Part model, mm, in its own coordinate system. Give positions to 0.01 mm unless a question says otherwise; leave off trailing zeros. Order: outer loops, then holes, each group sorted by start corner. A loop starts at its lowest first (then second) coordinate and runs counter-clockwise, first axis right, second up. Notation, with made-up numbers: (-18, -7.75) - (-10, -7.75) arc R15 cw to (-10, 18.25) - close; hole circle Ø6 at (66, 86). An arc over 180 degrees is marked (long way). One line per item, written item: value.
```python
from build123d import *
from OCP.BRepFilletAPI import BRepFilletAPI_MakeChamfer

# Parameters (mm, degrees)
BOSS_EXTRUDE1_DEPTH = 58.42
CHAMFER1_SIZE       = 6.35
CHAMFER1_SIZE2      = 6.020287439
CHAMFER1_SIZE2_2    = 11.16699707
CHAMFER2_SIZE       = 6.35
CHAMFER2_SIZE2      = 2.311210988
CHAMFER3_SIZE       = 6.35
CHAMFER3_SIZE_2     = 5.138982639
CHAMFER3_SIZE_3     = 2.835119985
CHAMFER3_SIZE_4     = 2.311210988


with BuildPart() as part:
    # Sketch1 → Boss-Extrude1 (new body)
    with BuildSketch(Plane(origin=(0, 0, 0), x_dir=(1, 0, 0), z_dir=(0, 1, 0))):
        with BuildLine():
            Line((-66.673768512, 0), (-37.067821873, 47.633329988))
            ThreePointArc((-37.067821873, 47.633329988), (-11.329209284, 68.541566023), (21.82652777, 69.113940477))
            Line((21.82652777, 69.113940477), (53.138492197, 58.903517294))
            Line((53.138492197, 58.903517294), (0, -77.45185891))
            Line((0, -77.45185891), (-66.673768512, -77.45185891))
            Line((-66.673768512, -77.45185891), (-66.673768512, 0))
        make_face()
    extrude(amount=BOSS_EXTRUDE1_DEPTH)

    # Chamfer1: one chamfer whose edges measure the first distance from different faces: ONE call of the kernel's chamfer builder (chamfer() names one face for all edges)
    chamfer1_edges_1 = [part.edges().sort_by_distance(p)[0] for p in [
        (26.569246099, 58.42, 9.274170808),
    ]]
    chamfer1_edges_2 = [part.edges().sort_by_distance(p)[0] for p in [
        (53.138492197, 29.21, -58.903517294),
    ]]
    chamfer1_side_2 = [part.faces().sort_by_distance(p)[0] for p in [
        (26.569246099, 29.21, 9.274170808),
    ]]
    chamfer1_edges_3 = [part.edges().sort_by_distance(p)[0] for p in [
        (0, 29.21, 77.45185891),
    ]]
    chamfer1_side_3 = [part.faces().sort_by_distance(p)[0] for p in [
        (-33.336884256, 29.21, 77.45185891),
    ]]
    chamfer1 = BRepFilletAPI_MakeChamfer(part.part.solid().wrapped)
    for e in chamfer1_edges_1:
        chamfer1.Add(CHAMFER1_SIZE, e.wrapped)
    for e in chamfer1_edges_2:
        chamfer1.Add(CHAMFER1_SIZE, CHAMFER1_SIZE2, e.wrapped, chamfer1_side_2[0].wrapped)  # the first distance lies on this face
    for e in chamfer1_edges_3:
        chamfer1.Add(CHAMFER1_SIZE, CHAMFER1_SIZE2_2, e.wrapped, chamfer1_side_3[0].wrapped)  # the first distance lies on this face
    add(Compound.cast(chamfer1.Shape()), mode=Mode.REPLACE)

    # Chamfer2
    chamfer2_edges = [part.edges().sort_by_distance(p)[0] for p in [
        (-36.744460568, 58.42, 77.45185891),
    ]]
    chamfer2_side = [part.faces().sort_by_distance(p)[0] for p in [
        (-36.512742561, 29.20916862, 77.45185891),
    ]]
    chamfer(chamfer2_edges, length=CHAMFER2_SIZE, length2=CHAMFER2_SIZE2, reference=chamfer2_side[0])

    # Chamfer3
    # the kernel refuses this chamfer: 6.35, 5.138982639, 2.835119985, 2.311210988 mm, written as the material it takes off along each edge
    with BuildSketch(Plane(origin=(53.073265581, 58.42, -76.224082144), x_dir=(0.6674738144333207, -0.6977227871251095, 0.2601184718012205), z_dir=(-0.3631074004698769, 0, 0.9317472917717596))) as chamfer3_piece_1:
        Polygon((CHAMFER3_SIZE * 0.999913086528, -CHAMFER3_SIZE * 0.0131840581986), (-CHAMFER3_SIZE_2 * 0.716367861072, -CHAMFER3_SIZE_2 * 0.69772278716), (0, 0), align=None)
    extrude(amount=178.925693595, mode=Mode.SUBTRACT)
    with BuildSketch(Plane(origin=(10.558676445, 58.42, 75.140647923), x_dir=(0, -0.9351017353626564, 0.3543793793687052), z_dir=(-1, 0, 0))) as chamfer3_piece_2:
        Polygon((CHAMFER3_SIZE * 0.999913086528, -CHAMFER3_SIZE * 0.0131840581986), (-CHAMFER3_SIZE_3 * 0.354379379374, -CHAMFER3_SIZE_3 * 0.935101735377), (0, 0), align=None)
    extrude(amount=93.705581509, mode=Mode.SUBTRACT)
    with BuildSketch(Plane(origin=(21.82652777, 58.42, -69.113940477), x_dir=(-0.3084963411353717, 0.09904090225204967, 0.946055446148474), z_dir=(0.9507298394814789, 0, 0.3100205998309168))) as chamfer3_piece_3:
        Polygon((CHAMFER3_SIZE_4 * 0.995083363005, CHAMFER3_SIZE_4 * 0.0990409022345), (-CHAMFER3_SIZE * 0.099040902252, CHAMFER3_SIZE * 0.995083363182), (0, 0), align=None)
    extrude(amount=43.047689039, mode=Mode.SUBTRACT)
    with BuildSketch(Plane(origin=(6.077481299, 58.42, -20.816864631), x_dir=(-0.849316991574707, 0, -0.5278831763018113), z_dir=(-0.5278831763018113, 0, 0.849316991574707))) as chamfer3_piece_4:
        Polygon((50.8 - CHAMFER3_SIZE_4, 0), (50.8, CHAMFER3_SIZE), (50.8, 0), align=None)
    revolve(axis=Axis((6.077481299, 58.42, -20.816864631), (0, -1, 0)), revolution_arc=76.197931096, mode=Mode.SUBTRACT)
    with BuildSketch(Plane(origin=(-75.369660158, 58.42, 13.990914778), x_dir=(0.8451412083835613, 0.0990409022520497, 0.5252877664414751), z_dir=(0.5278831763018161, 0, -0.849316991574704))) as chamfer3_piece_5:
        Polygon((CHAMFER3_SIZE_4 * 0.995083363005, CHAMFER3_SIZE_4 * 0.0990409022345), (-CHAMFER3_SIZE * 0.0990409022521, CHAMFER3_SIZE * 0.995083363182), (0, 0), align=None)
    extrude(amount=72.557414224, mode=Mode.SUBTRACT)
    with BuildSketch(Plane(origin=(-66.673768512, 58.42, 91.613784474), x_dir=(0.9950833631817486, 0.09904090225205003, 0), z_dir=(0, 0, -1))) as chamfer3_piece_6:
        Polygon((CHAMFER3_SIZE_4 * 0.995083363005, CHAMFER3_SIZE_4 * 0.0990409022345), (-CHAMFER3_SIZE * 0.0990409022521, CHAMFER3_SIZE * 0.995083363182), (0, 0), align=None)
    extrude(amount=108.086921026, mode=Mode.SUBTRACT)


solid = part.part
```
1) Slice it at A-A on y = 5. Write the cut outline in (x, z).
Answer:
outline: (-66.67, 0) - (-37.07, -47.63) arc R50.8 ccw to (21.83, -69.11) - (47.41, -60.77) - (50.83, -52.99) - (4.05, 67.05) - (-6.35, 77.45) - (-66.67, 77.45) - close
2) Wall check: line 1 along X through (y, z) = (13.5, -54.5); line 2 along Z through (x, y) = (-61, 7.5); line 3 along X through (y, z) = (15, 38). Give the ranges that are in metal, low to high. Write a range as [from, to].
Answer:
line 1: x = [-31.95, 50.17]
line 2: z = [-9.13, 77.45]
line 3: x = [-66.67, 15.37]
3) Slice it at B-B on z = 23. Write the cut outline in (x, y).
Answer:
outline: (-66.67, 0) - (21.22, 0) - (21.22, 52.07) - (19.22, 53.93) - (8.89, 58.42) - (-64.36, 58.42) - (-66.67, 52.07) - close
4) Slice it at C-C on x = -56. Write the cut outline in (y, z).
Answer:
outline: (0, -17.17) - (52.07, -17.17) - (58.42, -12.79) - (58.42, 72.31) - (52.45, 77.31) - (52.07, 77.45) - (0, 77.45) - close
